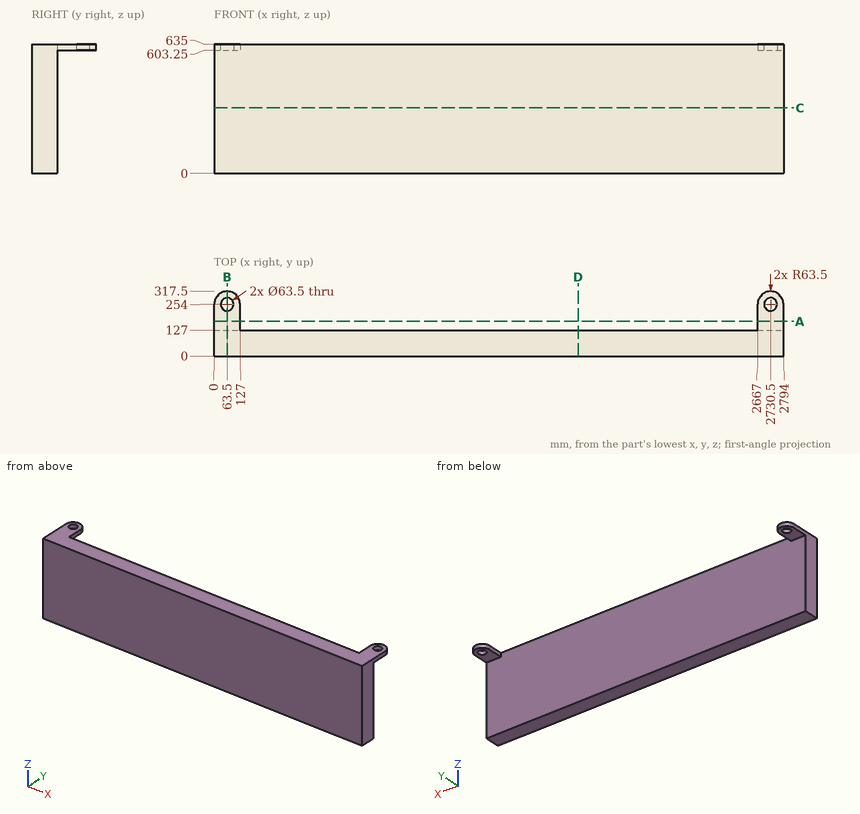
The drawing under review shows one solid part. Ordinate dimensions are in mm from its lowest x, y, z. Round coordinates to 2 decimals unless told otherwise and drop trailing zeros. Loops run counter-clockwise (first coordinate to the right, second up) from the corner with the lowest first, then second, coordinate; pieces in that order, holes last. Notation, with made-up numbers: (-6.5, 29.25) - (24.5, 29.25) arc R14 ccw to (24.5, 42.25) - close; hole circle Ø11 at (27.25, 84.25). An arc over 180 degrees is marked (long way). Use one line per item in the form item = value.
Item 1: Clearance check with a flat-ended pin moving along its axis: P1, Ø1.5, axis at x = 2354.5, z = 370, coming from the +Y side. State where the tip first meets the part, or that it passes through.
Answers:
P1 = 127
Item 2: Consider section B-B on x = 63.5. Write out the cut boundary in (y, z), then the cut area to 3 significant figures.
Answers:
outline = (0, 0) - (127, 0) - (127, 603.25) - (222.25, 603.25) - (222.25, 635) - (0, 635) - close; (285.75, 603.25) - (317.5, 603.25) - (317.5, 635) - (285.75, 635) - close
area = 84,700 mm^2
Item 3: Consider section A-A on y = 170.5. Write out the cut boundary in (x, z).
Answers:
outline = (0, 603.25) - (127, 603.25) - (127, 635) - (0, 635) - close; (2667, 603.25) - (2794, 603.25) - (2794, 635) - (2667, 635) - close
Item 4: Consider section C-C on z = 322. Write out the cut boundary in (x, y), then the cut area to 3 significant figures.
Answers:
outline = (0, 0) - (2794, 0) - (2794, 127) - (0, 127) - close
area = 355,000 mm^2
Item 5: Consider section D-D on x = 1786. Write out the cut boundary in (y, z), then the cut area to 3 significant figures.
Answers:
outline = (0, 0) - (127, 0) - (127, 635) - (0, 635) - close
area = 80,600 mm^2
Item 6: For line 1 (Y direction, x = 2730.5, z = 620); line 2 (Y direction, x = 1308.5, z = 511), list the stretches that pass through material, from the lowest coordinate up.
Answers:
line_1 = 0 to 222.25, 285.75 to 317.5
line_2 = 0 to 127
